```python
from build123d import *

# Parameters (mm, degrees)
BOSS_EXTRUDE1_START = 15.549813
SKETCH1_W           = 90
SKETCH1_H           = 100
SKETCH1_R           = 2.5
SKETCH1_R_2         = 3.57
BOSS_EXTRUDE1_DEPTH = 3.18
FILLET1_R           = 10


with BuildPart() as part:
    # Sketch1 → Boss-Extrude1 (new body)
    with BuildSketch(Plane.XY.offset(BOSS_EXTRUDE1_START)):
        with Locations((0, -5)):
            Rectangle(SKETCH1_W, SKETCH1_H)
        with Locations((32.3, -42.3)):
            Circle(SKETCH1_R, mode=Mode.SUBTRACT)
        with Locations((-32.3, -42.3)):
            Circle(SKETCH1_R_2, mode=Mode.SUBTRACT)
        with Locations((-32.3, 32.3)):
            Circle(SKETCH1_R_2, mode=Mode.SUBTRACT)
        with Locations((32.3, 32.3)):
            Circle(SKETCH1_R, mode=Mode.SUBTRACT)
    extrude(amount=BOSS_EXTRUDE1_DEPTH)

    # Fillet1
    fillet1_edges = [part.edges().sort_by_distance(p)[0] for p in [
        (-45, 45, 17.139813),
        (45, 45, 17.139813),
        (45, -55, 17.139813),
        (-45, -55, 17.139813),
    ]]
    fillet(fillet1_edges, radius=FILLET1_R)


solid = part.part
```
For this review, take the finished solid that the model builds, in its own axes (mm). Round coordinates to 2 decimals unless told otherwise and drop trailing zeros. Write each loop counter-clockwise with the first axis right and the second up, starting at its lowest first coordinate (ties: lowest second). Pieces come first, ordered by that corner, then holes. Notation, with made-up numbers: (50, 43.25) - (66, 43.25) arc R23 ccw to (66, 61.25) - close; hole circle Ø3 at (81, 30.5). An arc over 180 degrees is marked (long way). Answer as CSV lines item,"result". Start each with the question number.
(1) Add section C-C, the plane z = 17.15. State the section outline as (x, y) points.
(2) Add section A-A, the plane x = -32.3. State the section outline as (y, z) points, plus the area to 3 significant figures.
(3) Mouldability with a two-part tool opening along X and no side actions: class faces 1 (the cylindrical face through (-42.15, -51.99, 17.16)), 2 (the cylindrical face through (33.64, -40.19, 17.12)), 3 (the flat face through (0, 45, 17)) as +X half, -X half, draft (parallel to the pull), parting line (faces both ways), or undercut.
(4) For line 1 (Y direction, x = -32.3, z = 16.5); line 2 (Y direction, x = 32.3, z = 17.35); line 3 (X direction, y = -43, z = 18.45), list the stretches that pass through material, from the lowest coordinate up.
(5) Add section B-B, the plane y = 32.3. State the section outline as (x, z) points.
From the geometry:
1,outline,"(-45, -45) arc R10 ccw to (-35, -55) - (35, -55) arc R10 ccw to (45, -45) - (45, 35) arc R10 ccw to (35, 45) - (-35, 45) arc R10 ccw to (-45, 35) - close; hole circle Ø7.14 at (-32.3, -42.3); hole circle Ø7.14 at (-32.3, 32.3); hole circle Ø5 at (32.3, -42.3); hole circle Ø5 at (32.3, 32.3)"
2,outline,"(-55, 15.55) - (-45.87, 15.55) - (-45.87, 18.73) - (-55, 18.73) - close; (-38.73, 15.55) - (28.73, 15.55) - (28.73, 18.73) - (-38.73, 18.73) - close; (35.87, 15.55) - (45, 15.55) - (45, 18.73) - (35.87, 18.73) - close"
2,area,"273 mm²"
3,face 1,"-X half"
3,face 2,"undercut"
3,face 3,"draft"
4,line 1,"y = -55 to -45.87, -38.73 to 28.73, 35.87 to 45"
4,line 2,"y = -55 to -44.8, -39.8 to 29.8, 34.8 to 45"
4,line 3,"x = -45 to -35.8, -28.8 to 29.9, 34.7 to 45"
5,outline,"(-45, 15.55) - (-35.87, 15.55) - (-35.87, 18.73) - (-45, 18.73) - close; (-28.73, 15.55) - (29.8, 15.55) - (29.8, 18.73) - (-28.73, 18.73) - close; (34.8, 15.55) - (45, 15.55) - (45, 18.73) - (34.8, 18.73) - close"
